Model file for the job. Use its own axes, mm. A direction names the side the tool comes from. Coordinates: 2 decimals unless noted, no trailing zeros. Write each loop counter-clockwise with the first axis right and the second up, starting at its lowest first coordinate (ties: lowest second). Pieces come first, ordered by that corner, then holes. Notation, with made-up numbers: M 4.25,14 L 51.25,14 A18 ccw 51.25,38 Z; hole C 88,-22.75 d4. An arc over 180 degrees is marked long. Answer in a Markdown table with one row per item. Add a question column.
```python
from build123d import *

# Parameters (mm, degrees)
BOSS_EXTRUDE1_DEPTH = 6.35


with BuildPart() as part:
    # Sketch1 → Boss-Extrude1 (new body)
    with BuildSketch(Plane.XY):
        with BuildLine():
            Line((8.142065145, 0), (11.317065145, 0))
            Line((11.317065145, 0), (11.317065145, -6.35))
            Line((11.317065145, -6.35), (14.492065145, -6.35))
            Line((14.492065145, -6.35), (14.492065145, 0))
            Line((14.492065145, 0), (17.667065145, 0))
            Line((17.667065145, 0), (17.667065145, -6.35))
            Line((17.667065145, -6.35), (20.842065145, -6.35))
            Line((20.842065145, -6.35), (20.842065145, 0))
            Line((20.842065145, 0), (24.017065145, 0))
            Line((24.017065145, 0), (24.017065145, -6.35))
            Line((24.017065145, -6.35), (24.41861196, -6.35))
            ThreePointArc((24.41861196, -6.35), (27.024805452, -6.80954223), (29.316653546, -8.132741343))
            Line((29.316653546, -8.132741343), (35.829824373, -13.597940583))
            ThreePointArc((35.829824373, -13.597940583), (38.340167596, -15.241639353), (41.166077246, -16.250501778))
            ThreePointArc((41.166077246, -16.250501778), (42.360633111, -16.553938407), (43.539063258, -16.914964572))
            ThreePointArc((43.539063258, -16.914964572), (48.11077138, -16.040373561), (49.753251097, -11.685182984))
            Line((49.753251097, -11.685182984), (49.125880621, -7.532172023))
            Line((49.125880621, -7.532172023), (45.0441793, -12.396554237))
            Line((45.0441793, -12.396554237), (2.918629328, 22.950979207))
            Line((2.918629328, 22.950979207), (7.00033065, 27.815361421))
            Line((7.00033065, 27.815361421), (2.801471518, 27.712037944))
            ThreePointArc((2.801471518, 27.712037944), (-1.202340319, 25.338240278), (-1.269775543, 20.68411554))
            ThreePointArc((-1.269775543, 20.68411554), (1.266371651, 13.735078219), (1.692730633, 6.35))
            Line((1.692730633, 6.35), (8.142065145, 6.35))
            Line((8.142065145, 6.35), (8.142065145, 0))
        make_face()
    extrude(amount=BOSS_EXTRUDE1_DEPTH)


solid = part.part
```
1) Two-plate mould, pull along Y, no slides. Class faces 1 (the face through (38.3, -15.22, 3.13)), 2 (the face through (17.667, -3, 3)), 3 (the face through (4.93, 25.35, 3.13)): released by +Y, released by -Y, zero draft, split by the parting line, or undercut.
2) Flat gauge pins, fed straight in: pin 1 Ø1.9 at (y, z) = (-4.5, 2.5) entering from +X; pin 2 Ø2.5 at (x, z) = (10, 4) entering from -Y; pin 3 Ø3.5 at (x, z) = (19, 3) entering from -Y. Where does each tip first touch, or does it go through?
3) Which spindle directions (+Z, -Z, +X, -X, +Y, -Y) get a long thin tool onto all of the face, cutting with end or side? Do faces 4 (the face through (16, 0, 3)), 5 (the face through (19, -6.35, 3)), 6 (the face through (47.114, -9.93, 3.131)), 7 (the face through (1.245, 13.837, 3.131)). Say none if no direction does.
4) Slice it at C-C (x = 27). Give the cut face in (y, z).
5) Drill centre lines: probe 1 along X at (y, z) = (-10.5, 5); probe 2 along X at (y, z) = (-10, 6.25); probe 3 along X at (y, z) = (-13, 3.25). Where is each one in solid material? Low to high.
6) Slice it at D-D (y = 14). Give the cut face in (x, z).
7) Slice it at A-A (y = -10.5). Give the cut face in (x, z), then the cut area to 3 significant figures.
Ans:
| question | item | result |
|---|---|---|
| 1 | face 1 | released by -Y |
| 1 | face 2 | zero draft |
| 1 | face 3 | undercut |
| 2 | pin 1 | stops at x = 36.77 |
| 2 | pin 2 | stops at y = 0 |
| 2 | pin 3 | stops at y = -6.35 |
| 3 | face 4 | +Z, -Z, -Y |
| 3 | face 5 | +Z, -Z, -X, -Y |
| 3 | face 6 | +Z, -Z, +Y |
| 3 | face 7 | +Z, -Z, -X |
| 4 | outline | M -6.8,0 L 2.74,0 L 2.74,6.35 L -6.8,6.35 Z |
| 5 | probe 1 | x = 32.14 to 42.78, 46.64 to 49.57 |
| 5 | probe 2 | x = 31.54 to 42.19, 47.06 to 49.5 |
| 5 | probe 3 | x = 35.12 to 49.77 |
| 6 | outline | M 1.21,0 L 13.59,0 L 13.59,6.35 L 1.21,6.35 Z |
| 7 | outline | M 32.14,0 L 42.78,0 L 42.78,6.35 L 32.14,6.35 Z; M 46.64,0 L 49.57,0 L 49.57,6.35 L 46.64,6.35 Z |
| 7 | area | 86.3 mm2 |
